from build123d import *

# Parameters (mm, degrees)
SKETCH1_R      = 5
EXTRUDE1_DEPTH = 4
EXTRUDE4_START = 4.45086
EXTRUDE4_DEPTH = 7.205259
EXTRUDE5_START = 4.330127
EXTRUDE5_DEPTH = 7.205258
EXTRUDE6_START = 4.330127
EXTRUDE6_DEPTH = 7.205258


with BuildPart() as part:
    # Sketch1 → Extrude1 (new body)
    with BuildSketch(Plane(origin=(0, 0, 0), x_dir=(1, 0, 0), z_dir=(0, 1, 0))):
        with BuildLine():
            Line((-3.89089061, 3.146959138), (-2.360502052, 0.4962484))
            ThreePointArc((-2.360502052, 0.4962484), (-2.104118872, -0.718531203), (-2.613989574, -1.850544314))
            ThreePointArc((-2.613989574, -1.850544314), (-2.994220859, -5.370733384), (0.244467944, -6.801537968))
            ThreePointArc((0.244467944, -6.801537968), (1.479755407, -6.925983542), (2.403593813, -7.75540769))
            Line((2.403593813, -7.75540769), (3.933982371, -10.406118428))
            ThreePointArc((3.933982371, -10.406118428), (6.099045881, -11.656118428), (8.26410939, -10.406118428))
            Line((8.26410939, -10.406118428), (9.794497948, -7.75540769))
            ThreePointArc((9.794497948, -7.75540769), (10.718336354, -6.925983542), (11.953623817, -6.801537968))
            ThreePointArc((11.953623817, -6.801537968), (15.192312621, -5.370733384), (14.812081336, -1.850544314))
            ThreePointArc((14.812081336, -1.850544314), (14.302210633, -0.718531203), (14.558593813, 0.4962484))
            Line((14.558593813, 0.4962484), (16.088982371, 3.146959138))
            ThreePointArc((16.088982371, 3.146959138), (16.088982371, 5.646959138), (13.923918862, 6.896959138))
            Line((13.923918862, 6.896959138), (10.863141746, 6.896959138))
            ThreePointArc((10.863141746, 6.896959138), (9.68292016, 7.282314592), (8.9575034, 8.289882129))
            ThreePointArc((8.9575034, 8.289882129), (6.099045881, 10.379266616), (3.240588362, 8.289882129))
            ThreePointArc((3.240588362, 8.289882129), (2.515171602, 7.282314592), (1.334950016, 6.896959138))
            Line((1.334950016, 6.896959138), (-1.7258271, 6.896959138))
            ThreePointArc((-1.7258271, 6.896959138), (-3.89089061, 5.646959138), (-3.89089061, 3.146959138))
        make_face()
        with Locations((6.099045881, -0.120733384)):
            Circle(SKETCH1_R, mode=Mode.SUBTRACT)
    extrude(amount=EXTRUDE1_DEPTH)

    # GrooveSketch → Extrude4 (cut)
    with BuildSketch(Plane.XY.offset(EXTRUDE4_START)):
        Polygon((34.668922444, -26.069876563), (8.599045881, 0), (6.099045881, 2.5), (3.599045881, 0), (-22.470830682, -26.069876563), (-22.470830682, -99.806622573), (34.668922444, -99.806622573), align=None)
    extrude(amount=EXTRUDE4_DEPTH, mode=Mode.SUBTRACT)

    # Sketch9 → Extrude5 (cut)
    with BuildSketch(Plane(origin=(4.6265635, 0, 2.671147682), x_dir=(-0.5, 0, 0.866025404), z_dir=(-0.866025404, 0, -0.5)).offset(EXTRUDE5_START)):
        Polygon((32.223222882, -32.668187644), (-0.444964763, 0), (-2.944964763, 2.5), (-5.444964763, 0), (-38.113152407, -32.668187644), (-38.113152407, -125.067775694), (32.223222882, -125.067775694), align=None)
    extrude(amount=EXTRUDE5_DEPTH, mode=Mode.SUBTRACT)

    # Sketch10 → Extrude6 (cut)
    with BuildSketch(Plane(origin=(4.522005322, 0, -2.61078099), x_dir=(-0.5, 0, -0.866025404), z_dir=(0.866025404, 0, -0.5)).offset(EXTRUDE6_START)):
        Polygon((32.014106526, -32.668187644), (-0.654081118, 0), (-3.154081118, 2.5), (-5.654081118, 0), (-38.322268763, -32.668187644), (-38.322268763, -125.067775694), (32.014106526, -125.067775694), align=None)
    extrude(amount=EXTRUDE6_DEPTH, mode=Mode.SUBTRACT)


solid = part.part
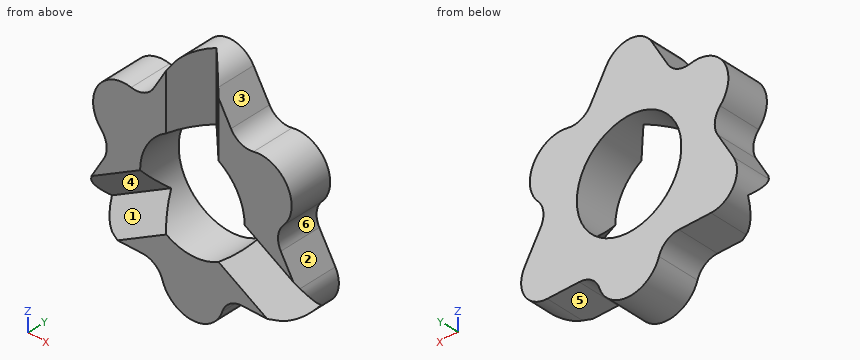
Input: part model. Units: mm. Frame: model coordinates. Face numbers are marked on the shaded views. A direction names the side the tool comes from. Round coordinates to 2 decimals unless told otherwise and drop trailing zeros. Order: outer loops, then holes, each group sorted by start corner. A loop starts at its lowest first (then second) coordinate and runs counter-clockwise, first axis right, second up. Notation, with made-up numbers: (85, 53) - (104, 53) arc R21 ccw to (104, 57) - close; hole circle Ø8 at (-39.75, -35). An arc over 180 degrees is marked (long way). Answer as a JSON object with one key per item and string values. Group by question number.
(1) Cut plane A-A (y = 0.6). Count the separate pieces of the cut face and the enclosed holes in it, then the cut area to 3 significant figures.
(2) Pin query (flat end, axial travel): P1, Ø0.9, axis at x = 0.5, y = 2.5, coming from the -Z side. Return the tip coordinate at first contact, or that it passes through.
(3) Cut plane C-C (z = 9.5). Return loops of the section in (x, y).
(4) Reachability of the marked faces 1, 2 and 3 from +Z, -Z, +X, -X, +Y, -Y: full face, straight path, thin tool, end or side. Return the list, or none.
(5) Material intervals for probe 1 along Z at (x, y) = (15, 3.75); probe 2 along Z at (x, y) = (-0.25, 1.5); probe 3 along Z at (x, y) = (-0.25, 3.1), sorted ascending. Write a range as from..to.
(6) Cut plane B-B (z = -4.5). Return loops of the section in (x, y).
(7) Draft query along X for the marked faces 4, 5 and 6. Return one class per face: released by +X, released by -X, zero draft, split by the parting line, or undercut.
Here are the results:
{
 "1": {"separate pieces": "3", "enclosed holes": "0", "area": "146 mm^2"},
 "2": {"P1": "stops at z = -6.9"},
 "3": {"outline": "(3.41, 0) - (3.6, 0) - (6.1, 2.5) - (8.6, 0) - (8.79, 0) - (8.79, 4) - (3.41, 4) - close"},
 "4": {"face 1": "-Y", "face 2": "+X, +Y, -Y", "face 3": "+Z, +X, +Y, -Y"},
 "5": {"probe 1": "z = -6.65..-1.26, 2.08..5.66", "probe 2": "z = -6.9..-4.7, -2.39..6.87", "probe 3": "z = -6.9..6.87"},
 "6": {"outline": "(-4.22, 1.34) - (-1.9, 2.5) - (3.1, 0) - (4.19, 0) - (4.19, 4) - (-4.22, 4) - close; (8.01, 0) - (9.1, 0) - (14.1, 2.5) - (16.42, 1.34) - (16.42, 4) - (8.01, 4) - close"},
 "7": {"face 4": "undercut", "face 5": "zero draft", "face 6": "released by +X"}
}
